Geometry: see drawing. Coordinates: mm, zero at the bounding-box minimum. Coordinates: 2 decimals unless noted, no trailing zeros. Loops run counter-clockwise (first coordinate to the right, second up) from the corner with the lowest first, then second, coordinate; pieces in that order, holes last. Notation, with made-up numbers: (65, 53) -> (124, 53) arc R20 cw to (124, 86) -> close; hole circle Ø1 at (-3, 25). An arc over 180 degrees is marked (long way). One line per item, written item: value. Start each with the question number.
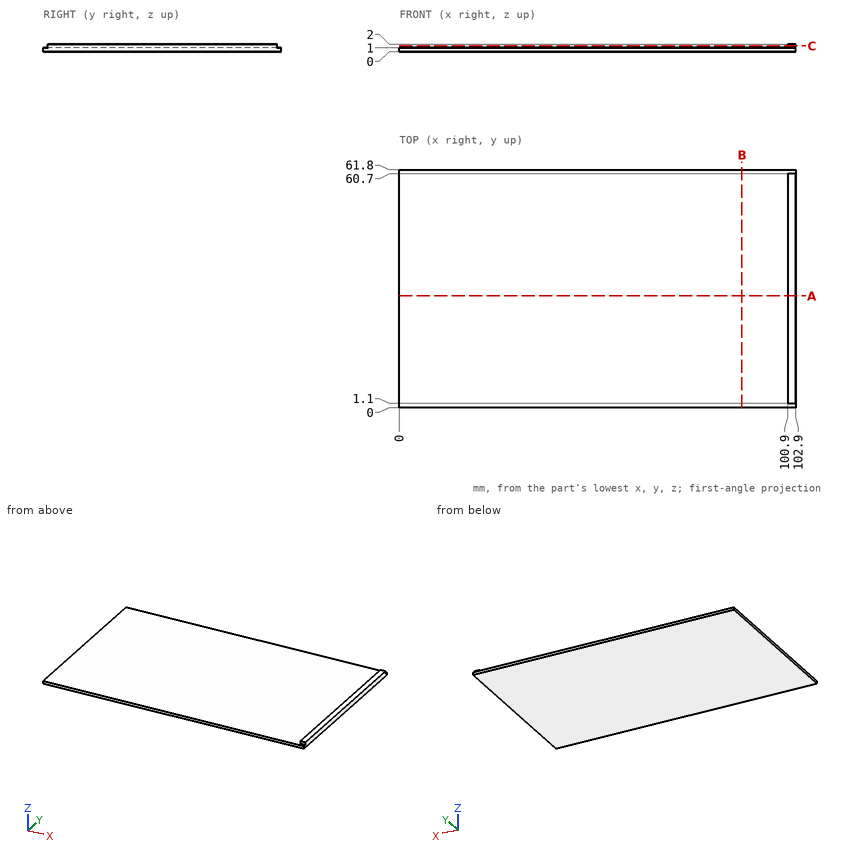
1. Line query: L1, parallel to Z at x = 26, y = 15.5; L2, parallel to X at y = 28.5, z = 1.5. Output: solid intervals per line, ascending. Write a range as [from, to].
2. Section C-C on z = 1.5. Return the cut outline in (x, y).
3. Section B-B on x = 89. Return the cut outline in (y, z), plus the area to 3 significant figures.
4. Section A-A on y = 29. Return the cut outline in (x, z).
5. Pin query (flat end, axial travel): pin 1 Ø1 at (x, y) = (81.5, 24) entering from +Z; pin 2 Ø0.8 at (y, z) = (21, 1.5) entering from -X. Return the tip coordinate at first contact, or that it passes through.
Checks:
1. L1: [0, 1]
1. L2: [100.9, 102.9]
2. outline: (100.9, 1.1) -> (102.9, 1.1) -> (102.9, 60.7) -> (100.9, 60.7) -> close
3. outline: (0, 0) -> (61.8, 0) -> (61.8, 1) -> (0, 1) -> close
3. area: 61.8 mm²
4. outline: (0, 0) -> (102.9, 0) -> (102.9, 2) -> (100.9, 2) -> (100.9, 1) -> (0, 1) -> close
5. pin 1: z = 1
5. pin 2: x = 100.9
